The model under review builds one solid part; all positions refer to its coordinate system, in mm. A direction names the side the tool comes from. Coordinates: 2 decimals unless noted, no trailing zeros. Write each loop counter-clockwise with the first axis right and the second up, starting at its lowest first coordinate (ties: lowest second). Pieces come first, ordered by that corner, then holes. Notation, with made-up numbers: (41, -12.5) - (59, -12.5) arc R23 cw to (59, 2.5) - close; hole circle Ø2 at (-37.5, -8.5). An arc over 180 degrees is marked (long way). Put each result on its own line as item: value. Start each with the question number.
Item 1: Mouldability with a two-part tool opening along Z and no side actions: class faces 4 (the face through (5, -33.5, 5)), 5 (the face through (6, -30, -4.2)), 6 (the face through (-7, -25.9, -4.2)), 7 (the face through (-2.38, 0.47, 10.74)) as pulls with the +Z half, pulls with the -Z half, needs draft (parallel to the pull), parting line crosses it, or undercut.
Item 2: Consider section A-A on z = 0. Give the boundary of the cut face in (x, y), then the cut area to 3 significant figures.
Item 3: Machinability: for faces 1 (the face through (-1.398, 33.993, 6.297)), 2 (the face through (0, -46.25, 0)), 3 (the face through (3, -34.5, -3)), which of the approach directions +Z, -Z, +X, -X, +Y, -Y give a long, thin tool a straight path to every point of the face, cutting with its end or side? Answer none if there is none.
Item 4: To check wall thickness, follow L1, parallel to Z at x = 0, y = -30; L2, parallel to Y at x = -8, z = -6.5; L3, parallel to Y at x = 5, z = 3. State the ranges of each line that lie inside material, in increasing order. Write a range as [from, to].
Item 5: Consider section B-B on x = -5. Give the boundary of the cut face in (y, z), then the cut area to 3 significant figures.
Item 6: For pin 1 (11 mm diameter, centred on x = -3, z = -5.5, fed in from -Y); pin 2 (1.5 mm diameter, centred on x = 7.25, z = -4.19, fed in from +Y); pin 3 (2 mm diameter, centred on x = -7.25, z = -4.19, fed in from -Y); pin 4 (6 mm diameter, centred on y = -20.5, z = -8.5, fed in from +X), all flat-tipped, find the tip position at first contact; note any pin that passes through.
Item 7: Consider section C-C on y = -8. Give the boundary of the cut face in (x, z), then the cut area to 3 significant figures.
```python
from build123d import *

# Parameters (mm, degrees)
SKETCH1_R                 = 11
BOSS_EXTRUDE1_DEPTH       = 33.5
SKETCH2_R                 = 6.45
BOSS_EXTRUDE2_DEPTH       = 1
SKETCH3_R                 = 6
BOSS_EXTRUDE3_DEPTH       = 1
SKETCH4_R                 = 3.25
BOSS_EXTRUDE4_DEPTH       = 1.5
SKETCH5_R                 = 2
BOSS_EXTRUDE5_DEPTH       = 10.25
M3X0_5_TAPPED_HOLE1_D     = 2.5
M3X0_5_TAPPED_HOLE1_DEPTH = 7
M3X0_5_TAPPED_HOLE1_TIP   = 0.751075774


with BuildPart() as part:
    # Sketch1 → Boss-Extrude1 (new body, symmetric)
    with BuildSketch(Plane(origin=(0, 0, 0), x_dir=(1, 0, 0), z_dir=(0, 1, 0))):
        Circle(SKETCH1_R)
    extrude(amount=BOSS_EXTRUDE1_DEPTH, both=True)

    # Sketch2 → Boss-Extrude2 (add)
    with BuildSketch(Plane(origin=(0, 33.5, 0), x_dir=(1, 0, 0), z_dir=(0, 1, 0))):
        Circle(SKETCH2_R)
    extrude(amount=BOSS_EXTRUDE2_DEPTH)

    # Sketch3 → Boss-Extrude3 (add)
    with BuildSketch(Plane.XZ.offset(33.5)):
        Circle(SKETCH3_R)
    extrude(amount=BOSS_EXTRUDE3_DEPTH)

    # Sketch4 → Boss-Extrude4 (add)
    with BuildSketch(Plane.XZ.offset(34.5)):
        Circle(SKETCH4_R)
    extrude(amount=BOSS_EXTRUDE4_DEPTH)

    # Sketch5 → Boss-Extrude5 (add)
    with BuildSketch(Plane(origin=(0, -36, 0), x_dir=(-1, 0, 0), z_dir=(0, -1, 0))):
        Circle(SKETCH5_R)
    extrude(amount=BOSS_EXTRUDE5_DEPTH)

    # M3x0.5 Tapped Hole1
    with Locations(Plane(origin=(0, -33.5, 0), x_dir=(-1, 0, 0), z_dir=(0, -1, 0))):
        with Locations((-7.25, 4.185631643), (7.25, 4.185631643), (0, -8.371736712)):
            Hole(M3X0_5_TAPPED_HOLE1_D / 2, depth=M3X0_5_TAPPED_HOLE1_DEPTH)
            with Locations((0, 0, -(M3X0_5_TAPPED_HOLE1_DEPTH + M3X0_5_TAPPED_HOLE1_TIP / 2))):  # 118° drill point
                Cone(0, M3X0_5_TAPPED_HOLE1_D / 2, M3X0_5_TAPPED_HOLE1_TIP, mode=Mode.SUBTRACT)


solid = part.part
```
Report:
1. face 4: needs draft
1. face 5: undercut
1. face 6: undercut
1. face 7: parting line crosses it
2. outline: (-11, -33.5) - (-6, -33.5) - (-6, -34.5) - (-3.25, -34.5) - (-3.25, -36) - (-2, -36) - (-2, -46.25) - (2, -46.25) - (2, -36) - (3.25, -36) - (3.25, -34.5) - (6, -34.5) - (6, -33.5) - (11, -33.5) - (11, 33.5) - (6.45, 33.5) - (6.45, 34.5) - (-6.45, 34.5) - (-6.45, 33.5) - (-11, 33.5) - close
2. area: 1,550 mm²
3. face 1: +Y
3. face 2: +Z, -Z, +X, -X, -Y
3. face 3: -Y
4. L1: [-11, 7.12], [9.62, 11]
4. L2: [-33.5, 33.5]
4. L3: [-34.5, 34.5]
5. outline: (-34.5, -3.32) - (-33.5, -3.32) - (-33.5, -9.8) - (33.5, -9.8) - (33.5, -4.07) - (34.5, -4.07) - (34.5, 4.07) - (33.5, 4.07) - (33.5, 9.8) - (-33.5, 9.8) - (-33.5, 3.32) - (-34.5, 3.32) - close
5. area: 1,330 mm²
6. pin 1: y = -46.25
6. pin 2: y = 33.5
6. pin 3: y = -26.35
6. pin 4: x = 9.53
7. outline: circle Ø22 at (0, 0)
7. area: 380 mm²
